The model under review builds one solid part; all positions refer to its coordinate system, in mm. Face numbers are marked on the shaded views. A direction names the side the tool comes from. Round coordinates to 2 decimals unless told otherwise and drop trailing zeros. Write each loop counter-clockwise with the first axis right and the second up, starting at its lowest first coordinate (ties: lowest second). Pieces come first, ordered by that corner, then holes. Notation, with made-up numbers: (0, 52.5) -> (5, 52.5) arc R16 ccw to (5, 60.5) -> close; hole circle Ø5 at (61, 7.25). An arc over 180 degrees is marked (long way). Return JSON: item names as keys, results as strings. Group by question number.
1. Take a section at A-A, the plane z = -56.5. Write out the cut boundary in (x, y) (1 decimal), then the cut area to 3 significant figures.
2. Take a section at D-D, the plane z = -40. Write out the cut boundary in (x, y), then the cut area to 3 significant figures.
3. Clearance check with flat-ended pins moving along their axes: P1, Ø3, axis at x = -11.5, y = 2.5, coming from the +Z side; P2, Ø1.9, axis at x = -43.5, y = 2.5, coming from the -Z side; P3, Ø18.5, axis at x = -35.5, z = -47.5, coming from the -Y side. State where each tip first meets the part, or that it passes through.
4. Tool access review of the marked faces 1 and 2: name each direction out of +Z, -Z, +X, -X, +Y, -Y from which nothing blocks a thin tool from reaching the whole face with its end or side.
5. For line 1 along Y through (x, z) = (-23.5, -85); line 2 along Z through (x, y) = (-41.5, 2.5); line 3 along X through (y, z) = (0.25, -72), list the stretches that pass through material, from the lowest coordinate up. Write a range as from..to.
6. Take a section at B-B, the plane y = 2.5. Write out the cut boundary in (x, z) (3 decimals), then the cut area to 3 significant figures.
7. Take a section at C-C, the plane x = -43. Write out the cut boundary in (y, z), then the cut area to 3 significant figures.
from build123d import *

# Parameters (mm, degrees)
F1_DEPTH  = 15.875
F2_W      = 4.318
F2_H      = 12.7
F3_DEPTH  = 9.175040233
F4_R      = 2.15899
F5_R      = 3.175
F6_DEPTH  = 3.81
F8_DEPTH  = 25.4
F10_DEPTH = 25.4


# Not quite as in the source:
# - a fillet or chamfer is up to 0.001 mm smaller than in the source, because OpenCascade refuses the exact size


with BuildPart() as f1:
    # F0 (on Front) → F1 (new body)
    with BuildSketch(Plane.XZ):
        Polygon((9.2045814112, -87.6168819653), (3.0183370735, -43.5994663098), (0, -44.0236659215), (6.1862443377, -88.041081577), align=None)
    extrude(amount=F1_DEPTH)

    # F2 (on face) → F3 (cut, through all)
    with BuildSketch(Plane(origin=(-6.067283434, 0, -0.8527010782), x_dir=(0, -1, 0), z_dir=(-0.9902680687, 0, -0.139173101))):
        with Locations((7.9375, -54.072730631)):
            Rectangle(F2_W, F2_H)
        with Locations((7.9375, -76.297730631)):
            Rectangle(F2_W, F2_H)
    extrude(amount=-F3_DEPTH, mode=Mode.SUBTRACT)

    # F4 (radius 2.159 in the source; OpenCascade refuses exactly that, so slightly less here)
    f4_edges = [f1.edges().sort_by_distance(p)[0] for p in [
        (2.083606, -5.7785, -47.898898),
        (5.176728, -5.7785, -69.907605),
        (5.176728, -10.0965, -69.907605),
        (2.083606, -10.0965, -47.898898),
        (3.851104, -10.0965, -60.475302),
        (6.944226, -10.0965, -82.48401),
        (6.944226, -5.7785, -82.48401),
        (3.851104, -5.7785, -60.475302),
    ]]
    fillet(f4_edges, radius=F4_R)

    # F5 (on Front) → F6 (join)
    with BuildSketch(Plane.XZ):
        Polygon((9.2045814112, -87.6168819653), (3.0183370735, -43.5994663098), (-19.3359767612, -43.5994663098), (-19.3359767612, -25.4), (-95.5359767612, -25.4), (-95.5359767612, -87.6168819653), align=None)
        with Locations((-82.8359767612, -34.925)):
            Circle(F5_R, mode=Mode.SUBTRACT)
    extrude(amount=-F6_DEPTH)

    # F7 (on Front) → F8 (cut)
    with BuildSketch(Plane.XZ):
        Polygon((-95.5359767612, -25.4), (-95.5359767612, -38.1), (-82.8359767612, -25.4), align=None)
    extrude(amount=-F8_DEPTH, mode=Mode.SUBTRACT)

    # F9 (on Front) → F10 (cut)
    with BuildSketch(Plane.XZ):
        Polygon((-70.1359767612, -23.5109585549), (-72.0250182062, -25.4), (-70.1359767612, -25.4), align=None)
        Polygon((-93.6469353161, -25.4), (-82.8359767612, -36.2109585549), (-72.0250182062, -25.4), align=None)
    extrude(amount=-F10_DEPTH, mode=Mode.SUBTRACT)


solid = f1.part
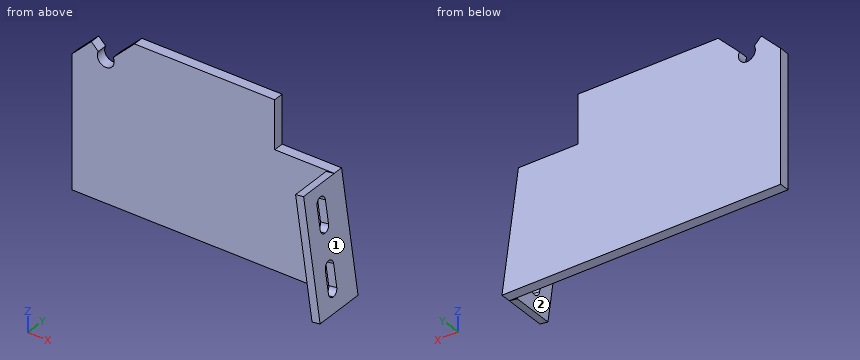
Output:
{
 "1": {"outline": "(-95.5, 0) -> (1.8, 0) -> (1.8, -5.8) -> (4.8, -5.8) -> (4.8, 3.8) -> (-95.5, 3.8) -> close; (1.8, -15.9) -> (4.8, -15.9) -> (4.8, -10.1) -> (1.8, -10.1) -> close", "area": "418 mm^2"},
 "2": {"outline": "(-95.54, 0) -> (-19.34, 0) -> (-19.34, 3.81) -> (-95.54, 3.81) -> close", "area": "290 mm^2"},
 "3": {"P1": "stops at z = -43.6", "P2": "stops at z = -87.62", "P3": "stops at y = 0"},
 "4": {"face 1": "+Z, +X, +Y, -Y", "face 2": "-Z, -X, -Y"},
 "5": {"line 1": "y = 0..3.81", "line 2": "z = -87.62..-25.4", "line 3": "x = -95.54..7.01"},
 "6": {"outline": "(-95.536, -87.617) -> (9.205, -87.617) -> (3.018, -43.599) -> (-19.336, -43.599) -> (-19.336, -25.4) -> (-72.025, -25.4) -> (-80.042, -33.417) arc R3.175 cw (long way) to (-85.63, -33.417) -> (-88.241, -30.805) -> (-95.536, -38.1) -> close", "area": "5,680 mm^2"},
 "7": {"outline": "(0, -87.62) -> (3.81, -87.62) -> (3.81, -25.4) -> (0, -25.4) -> close", "area": "237 mm^2"}
}
